Read the model definition and answer for the solid it produces. Units are mm, in the model's axes. Face numbers are marked on the shaded views. Coordinates: 2 decimals unless noted, no trailing zeros. Loops run counter-clockwise (first coordinate to the right, second up) from the corner with the lowest first, then second, coordinate; pieces in that order, holes last. Notation, with made-up numbers: (-23.5, -26.5) -> (-9.5, -26.5) arc R18 cw to (-9.5, -15.5) -> close; hole circle Ø8 at (-20, 41.25). An arc over 180 degrees is marked (long way). Answer in a Markdown table with one row per item.
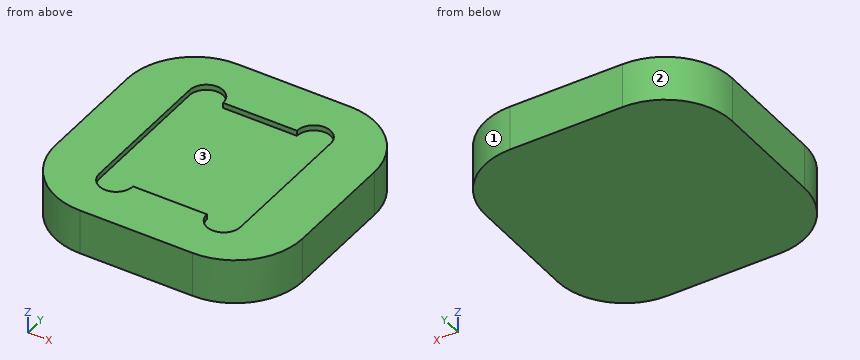
```python
from build123d import *

# Parameters (mm, degrees)
SKETCH1_W           = 35
SKETCH1_H           = 35
BOSS_EXTRUDE1_DEPTH = 6.35
CUT_EXTRUDE1_DEPTH  = 0.762
FILLET1_R           = 9.525


with BuildPart() as part:
    # Sketch1 → Boss-Extrude1 (new body)
    with BuildSketch(Plane.XY):
        Rectangle(SKETCH1_W, SKETCH1_H)
    extrude(amount=BOSS_EXTRUDE1_DEPTH)

    # Sketch3 → Cut-Extrude1 (cut)
    with BuildSketch(Plane.XY.offset(6.35)):
        with BuildLine():
            Line((-10, 10), (-10, -10))
            ThreePointArc((-10, -10), (-7.6124, -12.3876), (-5.2248, -10))
            Line((-5.2248, -10), (5.2248, -10))
            ThreePointArc((5.2248, -10), (7.6124, -12.3876), (10, -10))
            Line((10, -10), (10, 10))
            ThreePointArc((10, 10), (7.6124, 12.3876), (5.2248, 10))
            Line((5.2248, 10), (-5.2248, 10))
            ThreePointArc((-5.2248, 10), (-7.6124, 12.3876), (-10, 10))
        make_face()
    extrude(amount=-CUT_EXTRUDE1_DEPTH, mode=Mode.SUBTRACT)

    # Fillet1
    fillet1_edges = [part.edges().sort_by_distance(p)[0] for p in [
        (17.5, -17.5, 3.175),
        (-17.5, -17.5, 3.175),
        (-17.5, 17.5, 3.175),
        (17.5, 17.5, 3.175),
    ]]
    fillet(fillet1_edges, radius=FILLET1_R)


solid = part.part
```
1. A cutting plane is placed at A-A on z = 2.5. Give the vertices of the cut face in (x, y) (3 decimals), and give its area (3 significant figures).
A:
| item | result |
|---|---|
| outline | (-17.5, -7.975) arc R9.525 ccw to (-7.975, -17.5) -> (7.975, -17.5) arc R9.525 ccw to (17.5, -7.975) -> (17.5, 7.975) arc R9.525 ccw to (7.975, 17.5) -> (-7.975, 17.5) arc R9.525 ccw to (-17.5, 7.975) -> close |
| area | 1,150 mm2 |
2. A cutting plane is placed at C-C on y = 13.5. Give the vertices of the cut face in (x, z).
A:
| item | result |
|---|---|
| outline | (-15.73, 0) -> (15.73, 0) -> (15.73, 6.35) -> (-15.73, 6.35) -> close |
3. A cutting plane is placed at D-D on y = -13. Give the vertices of the cut face in (x, z).
A:
| item | result |
|---|---|
| outline | (-16.07, 0) -> (16.07, 0) -> (16.07, 6.35) -> (-16.07, 6.35) -> close |
4. The mould has two halves that part along X. Classify the marked faces 1, 2 and 3: pulls with the +X half, pulls with the -X half, needs draft (parallel to the pull), parting line crosses it, or undercut.
A:
| item | result |
|---|---|
| face 1 | pulls with the +X half |
| face 2 | pulls with the -X half |
| face 3 | undercut |
5. Find the intervals of material crossed by probe 1 along Y at (x, z) = (-1, 5.75); probe 2 along Z at (x, y) = (-3, -4.5); probe 3 along X at (y, z) = (13, 6), in increasing order.
A:
| item | result |
|---|---|
| probe 1 | y = -17.5 to -10, 10 to 17.5 |
| probe 2 | z = 0 to 5.59 |
| probe 3 | x = -16.07 to 16.07 |
6. A cutting plane is placed at B-B on x = 4.5. Give the vertices of the cut face in (y, z).
A:
| item | result |
|---|---|
| outline | (-17.5, 0) -> (17.5, 0) -> (17.5, 6.35) -> (10, 6.35) -> (10, 5.59) -> (-10, 5.59) -> (-10, 6.35) -> (-17.5, 6.35) -> close |
7. Given pin 1 Ø2 at (x, z) = (9.5, 5.5) entering from -Y; pin 2 Ø1.5 at (x, z) = (11.5, 1.5) entering from -Y; pin 3 Ø2 at (x, z) = (-13.5, 3.5) entering from +Y, each flat-ended and moving along its own axis, determine where each tip first touches the part or whether it passes through.
A:
| item | result |
|---|---|
| pin 1 | stops at y = -17.49 |
| pin 2 | stops at y = -17.09 |
| pin 3 | stops at y = 16.36 |
